from build123d import *

# Parameters (mm, degrees)
SKETCH1_R                = 69.85
BOSS_EXTRUDE1_DEPTH      = 7.62
SKETCH5_R                = 43.18
BOSS_EXTRUDE2_DEPTH      = 12.7
BOSS_EXTRUDE2_DEPTH_BACK = 14.1478
SKETCH6_R                = 1.190625
CUT_EXTRUDE2_DEPTH       = 17.3228
SKETCH7_R                = 38.1
CUT_EXTRUDE3_DEPTH       = 9.525


with BuildPart() as part:
    # Sketch1 → Boss-Extrude1 (new body)
    with BuildSketch(Plane(origin=(0, 0, 0), x_dir=(1, 0, 0), z_dir=(0, 1, 0))):
        Circle(SKETCH1_R)
    extrude(amount=BOSS_EXTRUDE1_DEPTH)

    # Sketch3 → Revolve1 (revolve)
    with BuildSketch(Plane.XY):
        Polygon((0, 14.1478), (31.873518738, 14.1478), (43.18, 7.62), (0, 7.62), align=None)
    revolve(axis=Axis((0, 7.62, 0), (0, 1, 0)))

    # Sketch5 → Boss-Extrude2 (add, two sides)
    with BuildSketch(Plane(origin=(0, 14.1478, 0), x_dir=(1, 0, 0), z_dir=(0, 1, 0))) as boss_extrude2_sk:
        Circle(SKETCH5_R)
    extrude(amount=BOSS_EXTRUDE2_DEPTH)
    extrude(boss_extrude2_sk.sketch, amount=-BOSS_EXTRUDE2_DEPTH_BACK)

    # Sketch6 → Cut-Extrude2 (cut)
    with BuildSketch(Plane(origin=(0, 26.8478, 0), x_dir=(1, 0, 0), z_dir=(0, 1, 0))):
        Circle(SKETCH6_R)
    extrude(amount=-CUT_EXTRUDE2_DEPTH, mode=Mode.SUBTRACT)

    # Sketch7 → Cut-Extrude3 (cut)
    with BuildSketch(Plane.XZ):
        Circle(SKETCH7_R)
    extrude(amount=-CUT_EXTRUDE3_DEPTH, mode=Mode.SUBTRACT)


solid = part.part
Part model, mm, in its own coordinate system. A direction names the side the tool comes from. Coordinates: 2 decimals unless noted, no trailing zeros. Order: outer loops, then holes, each group sorted by start corner. A loop starts at its lowest first (then second) coordinate and runs counter-clockwise, first axis right, second up. Notation, with made-up numbers: M -37.5,11.5 L -3.5,11.5 A13 cw -3.5,16.5 Z; hole C 25,11.5 d9. An arc over 180 degrees is marked long. Use a Markdown table: item, result.
(1) Cut at D-D on z = 40. Write the cut outline in (x, y).
A:
| item | result |
|---|---|
| outline | M -57.26,0 L 57.26,0 L 57.26,7.62 L 16.26,7.62 L 16.26,26.85 L -16.26,26.85 L -16.26,7.62 L -57.26,7.62 Z |
(2) Cut at A-A on y = 12. Write the cut outline in (x, z), then the cut area to 3 significant figures.
A:
| item | result |
|---|---|
| outline | C 0,0 d86.36; hole C 0,0 d2.38 |
| area | 5,850 mm^2 |
(3) Cut at C-C on z = -29. Write the cut outline in (x, y) (3 decimals), then the cut area to 3 significant figures.
A:
| item | result |
|---|---|
| outline | M -63.545,0 L -24.711,0 L -24.711,9.525 L 24.711,9.525 L 24.711,0 L 63.545,0 L 63.545,7.62 L 31.992,7.62 L 31.992,26.848 L -31.992,26.848 L -31.992,7.62 L -63.545,7.62 Z |
| area | 1,730 mm^2 |
(4) Flat gauge pins, fed straight in: pin 1 (3 mm diameter, centred on y = 6, z = 32.5, fed in from -X); pin 2 (3 mm diameter, centred on y = 7, z = 10, fed in from +X); pin 3 (5 mm diameter, centred on x = -33.5, y = 3, fed in from -Z). Where does each tip first touch, or does it go through?
A:
| item | result |
|---|---|
| pin 1 | stops at x = -62.59 |
| pin 2 | stops at x = 69.33 |
| pin 3 | stops at z = -62.59 |
(5) Probe L1, parallel to Z at x = 0, y = 15.5; L2, parallel to Y at x = 54, z = 30.5. List the from-to ranges inside material, lowest first.
A:
| item | result |
|---|---|
| L1 | z = -43.18 to -1.19, 1.19 to 43.18 |
| L2 | y = 0 to 7.62 |
(6) Pull direction Z, two halves, no side cores. Call faces 3 (the flat face through (-1, 26.848, 9)), 4 (the flat face through (8, 9.525, 1)), 5 (the cylindrical face through (-55.431, 3.757, 42.503)), 6 (the cylindrical face through (-30.235, 4.696, -23.183)): released by +Z, released by -Z, zero draft, split by the parting line, or undercut.
A:
| item | result |
|---|---|
| face 3 | zero draft |
| face 4 | undercut |
| face 5 | split by the parting line |
| face 6 | undercut |
(7) Cut at B-B on x = 6.5. Write the cut outline in (y, z) (3 decimals).
A:
| item | result |
|---|---|
| outline | M 0,-69.547 L 7.62,-69.547 L 7.62,-42.688 L 26.848,-42.688 L 26.848,42.688 L 7.62,42.688 L 7.62,69.547 L 0,69.547 L 0,37.541 L 9.525,37.541 L 9.525,-37.541 L 0,-37.541 Z |
(8) Tool access for faces 1 (the flat face through (30, 7.62, -32)), 2 (the flat face through (30, 0, 30)): list every direction of +Z, -Z, +X, -X, +Y, -Y with a clear straight run to the whole face (end or side of a thin tool).
A:
| item | result |
|---|---|
| face 1 | +Y |
| face 2 | +Z, -Z, +X, -X, -Y |
